Design review of the part built by this model. Coordinates are the model's own, in mm. A direction names the side the tool comes from. Give positions to 0.01 mm unless a question says otherwise; leave off trailing zeros. Loops run counter-clockwise (first coordinate to the right, second up) from the corner with the lowest first, then second, coordinate; pieces in that order, holes last. Notation, with made-up numbers: (-5, 58) -> (23, 58) arc R27 cw to (23, 87) -> close; hole circle Ø3 at (87.25, 48). An arc over 180 degrees is marked (long way). Answer in a Markdown table with one row per item. Add a question column.
(1) For pin 1 (1.2 mm diameter, centred on x = 14.5, z = 61.5, fed in from +Y); pin 2 (1 mm diameter, centred on y = 118, z = 63.5, fed in from -X); pin 3 (1.6 mm diameter, centred on y = 96.5, z = 64, fed in from +X), all flat-tipped, find the tip position at first contact; note any pin that passes through.
(2) Consider section B-B on y = 92.5. Write out the cut boundary in (x, z), then the cut area to 3 significant figures.
(3) For line 1 (X direction, y = 108.5, z = 64.95); line 2 (Y direction, x = 13.5, z = 60.4); line 3 (X direction, y = 121.5, z = 63.1), list the stretches that pass through material, from the lowest coordinate up.
(4) Draft analysis for pull direction X (two halves, no side actions). For faces 5 (the flat face through (-3, 85, 63)), 6 (the flat face through (12, 121, 63)), 7 (the cylindrical face through (12.99, 108.521, 60.675)), state which applies: +X half, -X half, draft (parallel to the pull), parting line (faces both ways), or undercut.
(5) For faces 1 (the flat face through (12, 110, 60.9)), 2 (the flat face through (14, 117, 63)), 3 (the flat face through (-14, 117, 63)), 4 (the flat face through (13, 107, 63)), list the 3-axis set-ups (+Z, -Z, +X, -X, +Y, -Y) from which the entire face can be reached by the end or side of a thin tool; tool diameter is ignored.
(6) Consider section A-A on x = 13.25. Write out the cut boundary in (y, z), then the cut area to 3 significant figures.
(7) Consider section C-C on z = 61.2. Write out the cut boundary in (x, y).
Solid Edge part; units mm, degrees
sketch "Sketch1" plane through (0, 0, 60.0575) normal (0, 0, 1) x (1, 0, 0)
  line L0 (12, 117) -> (16, 117)
  line L1 (16, 117) -> (16, 110)
  line L2 (10.5, 110) -> (16, 110)
  line L3 (10.5, 110) -> (10.5, 85)
  line L4 (10.5, 85) -> (-16, 85)
  line L5 (-16, 85) -> (-16, 117)
  line L6 (-16, 117) -> (-12, 117)
  line L7 (-12, 117) -> (-12, 125)
  line L8 (-12, 125) -> (12, 125)
  line L9 (12, 125) -> (12, 117)
extrude "Protrusion1" add sketch "Sketch1" along normal blind 5.2
sketch "Sketch2" plane through (13.25, 110, 62.5575) normal (0, -1, 0) x (1, 0, 0)
  circle A0 centre (0, 0.1) radius 2
extrude "ExtrudedProtrusion_3" add sketch "Sketch2" along normal blind 3
chamfer "Chamfer_1" distance 5 angle 12 1 edges at (0, 125, 65.2575) measured on face at (10.9867, 118.7333, 65.2575)
Values follow:
| question | item | result |
|---|---|---|
| 1 | pin 1 | y = 117 |
| 1 | pin 2 | x = -12 |
| 1 | pin 3 | x = 10.5 |
| 2 | outline | (-16, 60.06) -> (10.5, 60.06) -> (10.5, 65.26) -> (-16, 65.26) -> close |
| 2 | area | 138 mm2 |
| 3 | line 1 | -16 to 10.5 |
| 3 | line 2 | 110 to 117 |
| 3 | line 3 | -12 to 12 |
| 4 | face 5 | draft |
| 4 | face 6 | +X half |
| 4 | face 7 | undercut |
| 5 | face 1 | -Y |
| 5 | face 2 | +Z, -Z, +X, +Y |
| 5 | face 3 | +Z, -Z, -X, +Y |
| 5 | face 4 | +Z, -Z, +X, -Y |
| 6 | outline | (107, 60.66) -> (110, 60.66) -> (110, 60.06) -> (117, 60.06) -> (117, 65.26) -> (110, 65.26) -> (110, 64.66) -> (107, 64.66) -> close |
| 6 | area | 48.4 mm2 |
| 7 | outline | (-16, 85) -> (10.5, 85) -> (10.5, 110) -> (11.88, 110) -> (11.88, 107) -> (14.62, 107) -> (14.62, 110) -> (16, 110) -> (16, 117) -> (12, 117) -> (12, 125) -> (-12, 125) -> (-12, 117) -> (-16, 117) -> close |
